Input: part model. Units: mm. Frame: model coordinates. Face numbers are marked on the shaded views. A direction names the side the tool comes from. Round coordinates to 2 decimals unless told otherwise and drop trailing zeros. Loops run counter-clockwise (first coordinate to the right, second up) from the corner with the lowest first, then second, coordinate; pieces in that order, holes last.
(1) Access query for the marked faces 1 and 2. Directions: +Z, -Z, +X, -X, +Y, -Y. A direction counts if a zero-diameter tool reaches every point of the face in a straight line with its end or side. Return the directions, or none.
(2) Cut plane C-C, the plane y = -10. Output: boundary loops of the cut face in (x, z).
(3) Cut plane B-B, the plane z = 4.5. Output: boundary loops of the cut face in (x, y), and give its area (3 significant figures).
(4) Line query: line 1 (Y direction, x = -2.5, z = 2.5); line 2 (X direction, y = 7, z = 36); line 3 (Y direction, x = -8, z = 39). Output: solid intervals per line, ascending.
(5) Draft query along X for the marked faces 3, 4 and 5. Return one class per face: released by +X, released by -X, zero draft, split by the parting line, or undercut.
(6) Cut plane A-A, the plane x = 12.5. Output: boundary loops of the cut face in (y, z).
(7) First-contact query: pin 1 Ø5 at (x, y) = (-2.5, 8.5) entering from +Z. Flat tip, straight axial feed; report the tip coordinate or a pass-through.
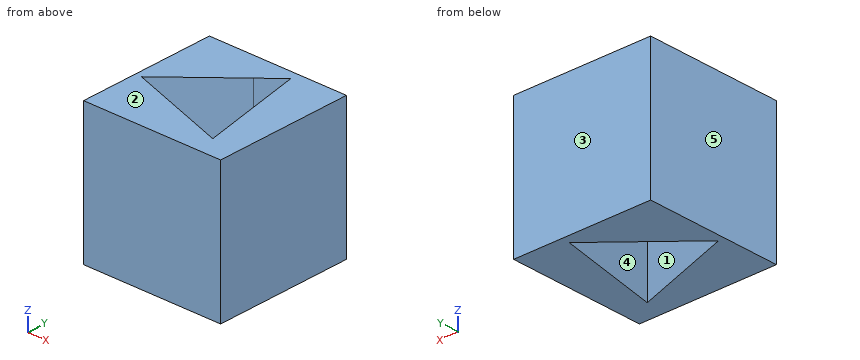
from build123d import *

# Parameters (mm, degrees)
F0_W     = 50
F0_H     = 50
F1_DEPTH = 50
F3_DEPTH = 55


with BuildPart() as f1:
    # F0 (on Top) → F1 (new body)
    with BuildSketch(Plane.XY):
        Rectangle(F0_W, F0_H)
    extrude(amount=F1_DEPTH)

    # F2 (on face) → F3 (cut)
    with BuildSketch(Plane.XY.offset(50)):
        Polygon((7.525486, 21.923712), (0, 15.369256), (-22.749234, -4.444594), (15.223748, -17.479118), align=None)
    extrude(amount=-F3_DEPTH, mode=Mode.SUBTRACT)


solid = f1.part
Reported:
1. face 1: +Z, -Z
1. face 2: +Z, +X, -X, +Y, -Y
2. outline: (-25, 0) - (-6.56, 0) - (-6.56, 50) - (-25, 50) - close; (13.76, 0) - (25, 0) - (25, 50) - (13.76, 50) - close
3. outline: (-25, -25) - (25, -25) - (25, 25) - (-25, 25) - close; hole (-22.75, -4.44) - (15.22, -17.48) - (7.53, 21.92) - close
3. area: 1,800 mm2
4. line 1: y = -25 to -11.4, 13.19 to 25
4. line 2: x = -25 to -9.61, 10.44 to 25
4. line 3: y = -25 to -9.51, 8.4 to 25
5. face 3: zero draft
5. face 4: undercut
5. face 5: released by -X
6. outline: (-25, 0) - (-16.54, 0) - (-16.54, 50) - (-25, 50) - close; (-3.54, 0) - (25, 0) - (25, 50) - (-3.54, 50) - close
7. pin 1: passes through
